Geometry: final body of the model. Coordinates: model frame, mm. Round coordinates to 2 decimals unless told otherwise and drop trailing zeros. Loops run counter-clockwise (first coordinate to the right, second up) from the corner with the lowest first, then second, coordinate; pieces in that order, holes last. Notation, with made-up numbers: M -35,21 L 21,21 A21 cw 21,45 Z; hole C 82,-31.5 d3. An arc over 180 degrees is marked long. Write each question's results on one line, items separated by ' | '.
```python
from build123d import *

# Parameters (mm, degrees)
SKETCH1_W                  = 50
SKETCH1_H                  = 40
BOSS_EXTRUDE1_DEPTH        = 3
M2_5_CLEARANCE_HOLE1_D     = 2.9
M2_5_CLEARANCE_HOLE1_DEPTH = 15.24
M2_5_CLEARANCE_HOLE1_TIP   = 0.871247898
M2_5_CLEARANCE_HOLE2_D     = 2.7
M2_5_CLEARANCE_HOLE2_DEPTH = 15.24
M2_5_CLEARANCE_HOLE2_TIP   = 0.811161836
FILLET1_R                  = 5


with BuildPart() as part:
    # Sketch1 → Boss-Extrude1 (new body)
    with BuildSketch(Plane(origin=(0, 0, 0), x_dir=(1, 0, 0), z_dir=(0, 1, 0))):
        with Locations((25, 20)):
            Rectangle(SKETCH1_W, SKETCH1_H)
    extrude(amount=BOSS_EXTRUDE1_DEPTH)

    # M2.5 Clearance Hole1
    with Locations(Plane(origin=(0, 3, 0), x_dir=(1, 0, 0), z_dir=(0, 1, 0))):
        with Locations((8.25, 35), (41.75, 35)):
            Hole(M2_5_CLEARANCE_HOLE1_D / 2, depth=M2_5_CLEARANCE_HOLE1_DEPTH)
            with Locations((0, 0, -(M2_5_CLEARANCE_HOLE1_DEPTH + M2_5_CLEARANCE_HOLE1_TIP / 2))):  # 118° drill point
                Cone(0, M2_5_CLEARANCE_HOLE1_D / 2, M2_5_CLEARANCE_HOLE1_TIP, mode=Mode.SUBTRACT)

    # M2.5 Clearance Hole2
    with Locations(Plane(origin=(0, 3, 0), x_dir=(1, 0, 0), z_dir=(0, 1, 0))):
        with Locations((3.5, 20), (46.5, 20)):
            Hole(M2_5_CLEARANCE_HOLE2_D / 2, depth=M2_5_CLEARANCE_HOLE2_DEPTH)
            with Locations((0, 0, -(M2_5_CLEARANCE_HOLE2_DEPTH + M2_5_CLEARANCE_HOLE2_TIP / 2))):  # 118° drill point
                Cone(0, M2_5_CLEARANCE_HOLE2_D / 2, M2_5_CLEARANCE_HOLE2_TIP, mode=Mode.SUBTRACT)

    # Fillet1
    fillet1_edges = [part.edges().sort_by_distance(p)[0] for p in [
        (0, 1.5, -40),
        (50, 1.5, -40),
        (50, 1.5, 0),
        (0, 1.5, 0),
    ]]
    fillet(fillet1_edges, radius=FILLET1_R)


solid = part.part
```
1. Pin query (flat end, axial travel): P1, Ø3.5, axis at x = 41.75, z = -35, coming from the +Y side. Return the tip coordinate at first contact, or that it passes through.
Answer key:
P1: stops at y = 3
2. Section B-B (z = -20). Output: boundary loops of the cut face in (x, y).
Answer key:
outline: M 0,0 L 2.15,0 L 2.15,3 L 0,3 Z; M 4.85,0 L 45.15,0 L 45.15,3 L 4.85,3 Z; M 47.85,0 L 50,0 L 50,3 L 47.85,3 Z
3. Section A-A (x = 8.25). Output: boundary loops of the cut face in (y, z).
Answer key:
outline: M 0,-40 L 3,-40 L 3,-36.45 L 0,-36.45 Z; M 0,-33.55 L 3,-33.55 L 3,0 L 0,0 Z
4. Draft query along X for faces 1 (the face through (47.85, 1.48, -20.06)), 2 (the face through (25, 1, -40)), 3 (the face through (48, 2, -39)). Return one class per face: pulls with the +X half, pulls with the -X half, needs draft (parallel to the pull), parting line crosses it, or undercut.
Answer key:
face 1: undercut | face 2: needs draft | face 3: pulls with the +X half
5. Section C-C (y = 1). Output: boundary loops of the cut face in (x, z), then the cut area to 3 significant figures.
Answer key:
outline: M 0,-35 A5 ccw 5,-40 L 45,-40 A5 ccw 50,-35 L 50,-5 A5 ccw 45,0 L 5,0 A5 ccw 0,-5 Z; hole C 3.5,-20 d2.7; hole C 8.25,-35 d2.9; hole C 41.75,-35 d2.9; hole C 46.5,-20 d2.7 | area: 1,950 mm²
6. Ray query, probe 1 along X at (y, z) = (1.3, -35); probe 2 along X at (y, z) = (1.4, -20); probe 3 along Z at (x, y) = (8.25, 2.1). Return the intervals inside material, ascending.
Answer key:
probe 1: x = 0 to 6.8, 9.7 to 40.3, 43.2 to 50 | probe 2: x = 0 to 2.15, 4.85 to 45.15, 47.85 to 50 | probe 3: z = -40 to -36.45, -33.55 to 0
7. Section D-D (z = -3). Output: boundary loops of the cut face in (x, y), then the cut area to 3 significant figures.
Answer key:
outline: M 0.42,0 L 49.58,0 L 49.58,3 L 0.42,3 Z | area: 147 mm²
